```python
from build123d import *

# Parameters (mm, degrees)
SKETCH1_W           = 40
SKETCH1_H           = 40
SKETCH1_R           = 2.5
BOSS_EXTRUDE1_DEPTH = 5
SKETCH2_R           = 16
BOSS_EXTRUDE2_DEPTH = 6
FILLET2_R           = 3


with BuildPart() as part:
    # Sketch1 → Boss-Extrude1 (new body)
    with BuildSketch(Plane.XY):
        Rectangle(SKETCH1_W, SKETCH1_H)
        with Locations((-15, 15)):
            Circle(SKETCH1_R, mode=Mode.SUBTRACT)
        with Locations((15, 15)):
            Circle(SKETCH1_R, mode=Mode.SUBTRACT)
        with Locations((15, -15)):
            Circle(SKETCH1_R, mode=Mode.SUBTRACT)
        with Locations((-15, -15)):
            Circle(SKETCH1_R, mode=Mode.SUBTRACT)
    extrude(amount=BOSS_EXTRUDE1_DEPTH)

    # Sketch2 → Boss-Extrude2 (add)
    with BuildSketch(Plane.XY.offset(5)):
        Circle(SKETCH2_R)
    extrude(amount=BOSS_EXTRUDE2_DEPTH)

    # Fillet2
    fillet2_edges = [part.edges().sort_by_distance(p)[0] for p in [
        (20, -20, 2.5),
        (-20, -20, 2.5),
        (-20, 20, 2.5),
        (20, 20, 2.5),
    ]]
    fillet(fillet2_edges, radius=FILLET2_R)


solid = part.part
```
Model file for the job. Use its own axes, mm. A direction names the side the tool comes from. Coordinates: 2 decimals unless noted, no trailing zeros. Loops run counter-clockwise (first coordinate to the right, second up) from the corner with the lowest first, then second, coordinate; pieces in that order, holes last. Notation, with made-up numbers: (40, 8.5) - (48, 8.5) arc R26 ccw to (48, 32.5) - close; hole circle Ø1 at (7, -15). An arc over 180 degrees is marked (long way). Answer as a JSON object with one key per item and string values. Group by question number.
(1) Probe line 1 along Y through (x, z) = (15, 4.25); line 2 along Y through (x, z) = (13.5, 3); line 3 along Z through (x, y) = (-9, -15). List the from-to ranges inside material, lowest first.
(2) Cut at B-B (x = -15). Give the cut face in (y, z).
(3) Cut at A-A (z = 1). Give the cut face in (x, y).
(4) Tool access for faces 1 (the face through (-9, 14, 5)), 2 (the face through (19.1, 19.14, 2.54)): list every direction of +Z, -Z, +X, -X, +Y, -Y with a clear straight run to the whole face (end or side of a thin tool).
(5) Flat gauge pins, fed straight in: pin 1 (4.5 mm diameter, centred on x = -15, y = 15, fed in from -Z); pin 2 (3 mm diameter, centred on x = 8, y = 4.5, fed in from -Z); pin 3 (1 mm diameter, centred on x = -5, z = 9, fed in from +Y); pin 4 (6.5 mm diameter, centred on x = 15, y = -15, fed in from +Z). Where does each tip first touch, or does it go through?
(6) Cut at D-D (x = 0). Give the cut face in (y, z), then the cut area to 3 significant figures.
(7) Two-plate mould, pull along X, no slides. Class faces 3 (the face through (-19.14, -19.1, 2.54)), 4 (the face through (12.5, -14.9, 2.5)), 5 (the face through (-17, -16.5, 2.5)), 6 (the face through (0, 0, 11)): released by +X, released by -X, zero draft, split by the parting line, or undercut.
(8) Cut at C-C (y = 14). Give the cut face in (x, z), then the cut area to 3 significant figures.
Geometry says:
{
 "1": {"line 1": "y = -20 to -17.5, -12.5 to 12.5, 17.5 to 20", "line 2": "y = -20 to -17, -13 to 13, 17 to 20", "line 3": "z = 0 to 5"},
 "2": {"outline": "(-20, 0) - (-17.5, 0) - (-17.5, 5) - (-20, 5) - close; (-12.5, 0) - (12.5, 0) - (12.5, 5) - (5.57, 5) - (5.57, 11) - (-5.57, 11) - (-5.57, 5) - (-12.5, 5) - close; (17.5, 0) - (20, 0) - (20, 5) - (17.5, 5) - close"},
 "3": {"outline": "(-20, -17) arc R3 ccw to (-17, -20) - (17, -20) arc R3 ccw to (20, -17) - (20, 17) arc R3 ccw to (17, 20) - (-17, 20) arc R3 ccw to (-20, 17) - close; hole circle Ø5 at (-15, -15); hole circle Ø5 at (-15, 15); hole circle Ø5 at (15, -15); hole circle Ø5 at (15, 15)"},
 "4": {"face 1": "+Z", "face 2": "+Z, -Z, +X, +Y"},
 "5": {"pin 1": "passes through", "pin 2": "stops at z = 0", "pin 3": "stops at y = 15.35", "pin 4": "stops at z = 5"},
 "6": {"outline": "(-20, 0) - (20, 0) - (20, 5) - (16, 5) - (16, 11) - (-16, 11) - (-16, 5) - (-20, 5) - close", "area": "392 mm^2"},
 "7": {"face 3": "released by -X", "face 4": "undercut", "face 5": "undercut", "face 6": "zero draft"},
 "8": {"outline": "(-20, 0) - (-17.29, 0) - (-17.29, 5) - (-20, 5) - close; (-12.71, 0) - (12.71, 0) - (12.71, 5) - (7.75, 5) - (7.75, 11) - (-7.75, 11) - (-7.75, 5) - (-12.71, 5) - close; (17.29, 0) - (20, 0) - (20, 5) - (17.29, 5) - close", "area": "247 mm^2"}
}
